Could you check a few things on this model? Use its own coordinates, in mm. A direction names the side the tool comes from. Coordinates: 2 decimals unless noted, no trailing zeros. Loops run counter-clockwise (first coordinate to the right, second up) from the corner with the lowest first, then second, coordinate; pieces in that order, holes last.
from build123d import *

# Parameters (mm, degrees)
SKETCH1_R           = 32
SKETCH1_R_2         = 22.5
SKETCH4_R           = 60
SKETCH4_R_2         = 22.5
BOSS_EXTRUDE1_DEPTH = 20
BOSS_EXTRUDE2_START = -20
SKETCH5_R           = 60
SKETCH5_R_2         = 22.5
BOSS_EXTRUDE2_DEPTH = 20
HOLE1_D             = 15
HOLE1_DEPTH         = 20
CIRPATTERN1_COUNT   = 4
HOLE2_D             = 15
HOLE2_DEPTH         = 20
CIRPATTERN2_COUNT   = 4
SKETCH10_R          = 12
BOSS_EXTRUDE3_DEPTH = 20
BOSS_EXTRUDE4_DEPTH = 12
SKETCH13_W          = 130
SKETCH13_H          = 64
BOSS_EXTRUDE6_DEPTH = 10


with BuildPart() as part:
    # Sweep1: sweep along a path in Sketch3
    with BuildLine(Plane(origin=(0, 0, 0), x_dir=(0, 0, -1), z_dir=(1, 0, 0))) as sweep1_path:
        Line((0, 0), (125, 0))
        ThreePointArc((125, 0), (158.941125497, 14.058874503), (173, 48))
        Line((173, 48), (173, 248))
    # Sketch1 → Sweep1 (sweep)
    with BuildSketch(Plane.XY):
        Circle(SKETCH1_R)
        Circle(SKETCH1_R_2, mode=Mode.SUBTRACT)
    sweep(path=sweep1_path.line)

    # Sketch4 → Boss-Extrude1 (add)
    with BuildSketch(Plane(origin=(0, 248, 0), x_dir=(1, 0, 0), z_dir=(0, 1, 0))):
        with Locations(Location((0, 173, 0), (0, 0, 270))):
            Circle(SKETCH4_R)
        with Locations((0, 173)):
            Circle(SKETCH4_R_2, mode=Mode.SUBTRACT)
    extrude(amount=-BOSS_EXTRUDE1_DEPTH)

    # Sketch5 → Boss-Extrude2 (add)
    with BuildSketch(Plane.XY.offset(BOSS_EXTRUDE2_START)):
        Circle(SKETCH5_R)
        with Locations(Location((0, 0, 0), (0, 0, 270))):
            Circle(SKETCH5_R_2, mode=Mode.SUBTRACT)
    extrude(amount=BOSS_EXTRUDE2_DEPTH)

    # Hole1
    with Locations(Plane.XY):
        with Locations((45, 0)):
            hole1 = Hole(HOLE1_D / 2, depth=HOLE1_DEPTH)

    # CirPattern1: Hole1 ×4 about axis
    cirpattern1_axis = Axis((0, 0, 0), (0, 0, 1))
    for i in range(1, CIRPATTERN1_COUNT):
        add(hole1.rotate(cirpattern1_axis, i * 360 / CIRPATTERN1_COUNT), mode=Mode.SUBTRACT)

    # Hole2
    with Locations(Plane(origin=(0, 248, 0), x_dir=(1, 0, 0), z_dir=(0, 1, 0))):
        with Locations((45, 173)):
            hole2 = Hole(HOLE2_D / 2, depth=HOLE2_DEPTH)

    # CirPattern2: Hole2 ×4 about axis
    cirpattern2_axis = Axis((0, 0, -173), (0, 1, 0))
    for i in range(1, CIRPATTERN2_COUNT):
        add(hole2.rotate(cirpattern2_axis, i * 360 / CIRPATTERN2_COUNT), mode=Mode.SUBTRACT)



with BuildPart() as body_2:
    # Sketch10 → Boss-Extrude3 (new body)
    with BuildSketch(Plane.XY.offset(-340)):
        with BuildLine():
            Line((-99.857142857, 195.852940773), (-10.714285714, 217.705881545))
            ThreePointArc((-10.714285714, 217.705881545), (0, 219), (10.714285714, 217.705881545))
            Line((10.714285714, 217.705881545), (99.857142857, 195.852940773))
            ThreePointArc((99.857142857, 195.852940773), (117, 174), (99.857142857, 152.147059227))
            Line((99.857142857, 152.147059227), (10.714285714, 130.294118455))
            ThreePointArc((10.714285714, 130.294118455), (0, 129), (-10.714285714, 130.294118455))
            Line((-10.714285714, 130.294118455), (-99.857142857, 152.147059227))
            ThreePointArc((-99.857142857, 152.147059227), (-117, 174), (-99.857142857, 195.852940773))
        make_face()
        with Locations((-94.5, 174)):
            Circle(SKETCH10_R, mode=Mode.SUBTRACT)
        with Locations((94.5, 174)):
            Circle(SKETCH10_R, mode=Mode.SUBTRACT)
    extrude(amount=BOSS_EXTRUDE3_DEPTH)


with BuildPart() as part_1:
    add(part.part)

    add(body_2.part)  # Boss-Extrude4 merges body 2
    # Sketch12 → Boss-Extrude4 (add, symmetric)
    with BuildSketch(Plane(origin=(0, 174, 0), x_dir=(1, 0, 0), z_dir=(0, 1, 0))):
        with BuildLine():
            Line((-31.562633586, 167.727414188), (-57, 320))
            Line((-57, 320), (57, 320))
            Line((57, 320), (31.562633586, 167.727414188))
            ThreePointArc((31.562633586, 167.727414188), (0, 205), (-31.562633586, 167.727414188))
        make_face()
    extrude(amount=BOSS_EXTRUDE4_DEPTH, both=True)

    # Sketch13 → Boss-Extrude6 (add, symmetric)
    with BuildSketch(Plane(origin=(0, 0, 0), x_dir=(0, 0, -1), z_dir=(1, 0, 0))):
        with Locations((261, 174)):
            Rectangle(SKETCH13_W, SKETCH13_H)
    extrude(amount=BOSS_EXTRUDE6_DEPTH, both=True)


solid = part_1.part
(1) I need wall thicknesses on probe 1 along Z at (x, y) = (0, 101); probe 2 along Y at (x, z) = (-29, -205); probe 3 along Y at (x, z) = (94.5, -327). Which ranges of each line are inside material? Lowest first, please.
Answers:
probe 1: z = -205 to -195.5, -150.5 to -141
probe 2: y = 162 to 186, 228 to 248
probe 3: y = 150.83 to 162, 186 to 197.17
(2) Imagine slicing it at B-B, the plane x = -94.5. Write out the boundary of the cut face in (y, z), and give its area (3 significant figures).
Answers:
outline: (150.83, -340) - (162, -340) - (162, -320) - (150.83, -320) - close; (186, -340) - (197.17, -340) - (197.17, -320) - (186, -320) - close
area: 447 mm2
(3) Imagine slicing it at A-A, the plane z = -218. Write out the boundary of the cut face in (x, y).
Answers:
outline: (-39.96, 162) - (-10, 162) - (-10, 142) - (10, 142) - (10, 162) - (39.96, 162) - (39.96, 186) - (10, 186) - (10, 206) - (-10, 206) - (-10, 186) - (-39.96, 186) - close; (-39.69, 228) - (-7.5, 228) - (-7.5, 248) - (-39.69, 248) - close; (7.5, 228) - (39.69, 228) - (39.69, 248) - (7.5, 248) - close
(4) Imagine slicing it at D-D, the plane x = 45. Write out the boundary of the cut face in (y, z), and give its area (3 significant figures).
Answers:
outline: (-39.69, -20) - (-7.5, -20) - (-7.5, 0) - (-39.69, 0) - close; (7.5, -20) - (39.69, -20) - (39.69, 0) - (7.5, 0) - close; (138.7, -340) - (209.3, -340) - (209.3, -320) - (186, -320) - (186, -248.17) - (162, -248.17) - (162, -320) - (138.7, -320) - close; (228, -212.69) - (248, -212.69) - (248, -180.5) - (228, -180.5) - close; (228, -165.5) - (248, -165.5) - (248, -133.31) - (228, -133.31) - close
area: 5,710 mm2
(5) Which directions (+Z, -Z, +X, -X, +Y, -Y) give clear straight access to the entire face, cutting with the end or side of a thin tool? Please do faces 4 (the face through (2.64, 238.14, -232.94)), 5 (the face through (44.46, 174.17, -244.93)), 6 (the face through (-54.662, 141.068, -330.14)).
Answers:
face 4: +Y
face 5: +Z, +X, -Y
face 6: -Z, -X, -Y
(6) For pin 1 (3 mm diameter, centred on y = 29, z = -127, fed in from +X); pin 2 (22 mm diameter, centred on y = 198.5, z = -289.5, fed in from +X); pin 3 (22 mm diameter, centred on y = 152.5, z = -264, fed in from +X); pin 4 (13.5 mm diameter, centred on x = 45, y = 0, fed in from -Z), each with a flat end and sliding along its axis, tell me the tip position at first contact or that it passes through.
Answers:
pin 1: stops at x = 16.54
pin 2: stops at x = 10
pin 3: stops at x = 48.57
pin 4: passes through
(7) We'd pull the mould along Y, two halves only. Please class faces 1 (the face through (85.656, 182.11, -330.14)), 2 (the face through (0, 219, -330)), 3 (the face through (-59.94, 2.64, -10.14)): +Y half, -Y half, draft (parallel to the pull), parting line (faces both ways), or undercut.
Answers:
face 1: undercut
face 2: +Y half
face 3: parting line
(8) Imagine slicing it at C-C, the plane y = 0. State how many separate pieces and enclosed holes the cut face has, and give its area (3 significant figures).
Answers:
separate pieces: 3
enclosed holes: 0
area: 4,400 mm2
